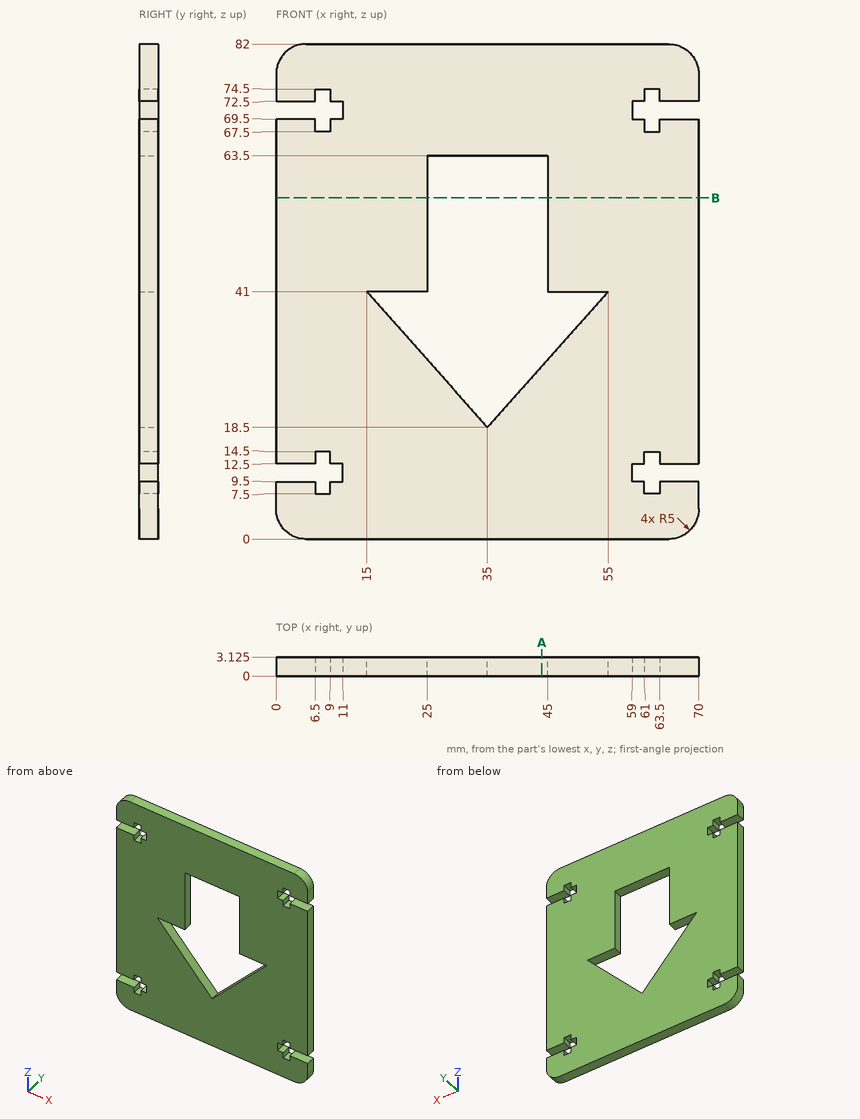
Geometry check sheet. Reference: drawing and pictorial views, mm from the part's lowest x, y, z. Give positions to 0.01 mm unless a question says otherwise; leave off trailing zeros. Order: outer loops, then holes, each group sorted by start corner. A loop starts at its lowest first (then second) coordinate and runs counter-clockwise, first axis right, second up. Notation, with made-up numbers: (39, -34) - (52, -34) arc R20 cw to (52, -15) - close; hole circle Ø10 at (62, 70). An arc over 180 degrees is marked (long way). Use one line per item in the form item = value.
1) Sectioned sample at A-A (x = 44). Record the boundary of the cut face in (y, z) (3 decimals).
Working result:
outline = (0, 0) - (3.125, 0) - (3.125, 28.625) - (0, 28.625) - close; (0, 63.5) - (3.125, 63.5) - (3.125, 82) - (0, 82) - close
2) Sectioned sample at B-B (z = 56.5). Record the boundary of the cut face in (x, y) (3 decimals).
Working result:
outline = (0, 0) - (25, 0) - (25, 3.125) - (0, 3.125) - close; (45, 0) - (70, 0) - (70, 3.125) - (45, 3.125) - close
3) Material ranges on probe 1 along Z at (x, y) = (7.5, 1.1); probe 2 along X at (y, z) = (1.35, 51); probe 3 along X at (y, z) = (1, 70), recorded low to high. Write a range as from..to.
Working result:
probe_1 = 0..7.5, 14.5..67.5, 74.5..82
probe_2 = 0..25, 45..70
probe_3 = 11..59
